from build123d import *

# Parameters (mm, degrees)
SCHIZZO1_W                   = 130
SCHIZZO1_H                   = 48.5
ESTRUSIONE_ESTRUSIONE1_DEPTH = 1.45
TAGLIO_ESTRUSIONE1_DEPTH     = 12
RACCORDO1_R                  = 1


with BuildPart() as part:
    # Schizzo1 → Estrusione-Estrusione1 (new body)
    with BuildSketch(Plane.XY):
        with Locations((65, 24.25)):
            Rectangle(SCHIZZO1_W, SCHIZZO1_H)
    extrude(amount=ESTRUSIONE_ESTRUSIONE1_DEPTH)

    # Schizzo2 → Taglio-Estrusione1 (cut)
    with BuildSketch(Plane.XY.offset(1.45)):
        with BuildLine():
            Line((144.922454277, 4.622930456), (115.077545723, 4.622930456))
            ThreePointArc((115.077545723, 4.622930456), (111.052124488, 8.64835169), (115.077545723, 12.673772925))
            Line((115.077545723, 12.673772925), (144.922454277, 12.673772925))
            ThreePointArc((144.922454277, 12.673772925), (148.947875512, 8.64835169), (144.922454277, 4.622930456))
        make_face()
    extrude(amount=-TAGLIO_ESTRUSIONE1_DEPTH, mode=Mode.SUBTRACT)

    # Raccordo1
    raccordo1_edges = [part.edges().sort_by_distance(p)[0] for p in [
        (130, 4.622930456, 0.725),
        (130, 12.673772925, 0.725),
        (0, 48.5, 0.725),
        (130, 48.5, 0.725),
        (130, 0, 0.725),
        (0, 0, 0.725),
    ]]
    fillet(raccordo1_edges, radius=RACCORDO1_R)


solid = part.part
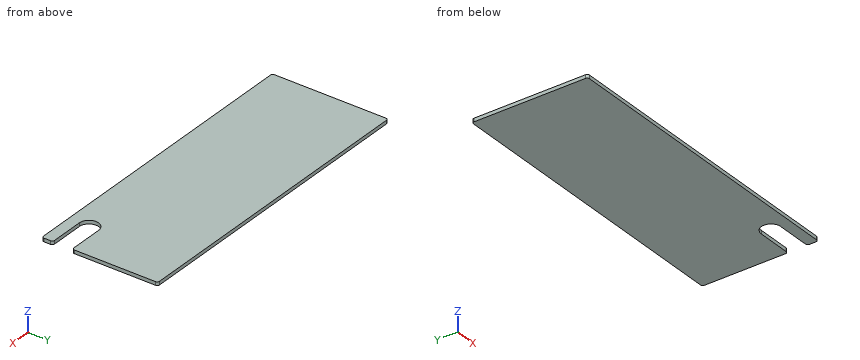
Source: CAD feature listing. Evaluate the final solid. Frame: model axes, mm. Round coordinates to 2 decimals unless told otherwise and drop trailing zeros. Loops run counter-clockwise (first coordinate to the right, second up) from the corner with the lowest first, then second, coordinate; pieces in that order, holes last.
Q1. First-contact query: P1, Ø4, axis at x = 29.5, y = 32.5, coming from the -Z side. Flat tip, straight axial feed; report the tip coordinate or a pass-through.
Q2. Section B-B, the plane y = 8.5. Return loops of the section in (x, z), plus the area to 3 significant figures.
Q3. Ray query, line 1 (X direction, y = 11.5, z = 0.35); line 2 (X direction, y = 10, z = 0.3). Return the intervals inside material, ascending.
Q4. Section A-A, the plane z = 0.3. Return loops of the section in (x, y).
Solutions:
1. P1: stops at z = 0
2. outline: (0, 0) - (111.05, 0) - (111.05, 1.45) - (0, 1.45) - close
2. area: 161 mm2
3. line 1: x = 0 to 112.24
3. line 2: x = 0 to 111.29
4. outline: (0, 1) arc R1 ccw to (1, 0) - (129, 0) arc R1 ccw to (130, 1) - (130, 3.62) arc R1 ccw to (129, 4.62) - (115.08, 4.62) arc R4.03 cw to (115.08, 12.67) - (129, 12.67) arc R1 ccw to (130, 13.67) - (130, 47.5) arc R1 ccw to (129, 48.5) - (1, 48.5) arc R1 ccw to (0, 47.5) - close
